Autodesk Fusion 360 part; units mm, degrees
sketch "Sketch1" plane through (0, 0, 0) normal (0, 0, 1) x (1, 0, 0)
  line L0 (0, 0) -> (55, 0)
  line L1 (55, 0) -> (55, 55)
  line L2 (55, 55) -> (0, 55)
  line L3 (0, 55) -> (0, 0)
  circle A0 centre (4, 51) radius 4
  circle A1 centre (51, 51) radius 4
  circle A2 centre (4, 4) radius 4
  circle A3 centre (51, 4) radius 4
  circle A4 centre (4, 51) radius 1.55
  circle A5 centre (51, 51) radius 1.55
  circle A6 centre (4, 4) radius 1.55
  circle A7 centre (51, 4) radius 1.55
  dimension "d1" = 55
  dimension "d2" = 55
  dimension "d3" = 8
  dimension "d4" = 8
  dimension "d5" = 8
  dimension "d6" = 8
  dimension "d7" = 4
  dimension "d8" = 4
  dimension "d9" = 4
  dimension "d10" = 4
  dimension "d11" = 4
  dimension "d12" = 4
  dimension "d13" = 4
  dimension "d14" = 4
  dimension "d15" = 3.1
  dimension "d16" = 3.1
  dimension "d17" = 3.1
  dimension "d18" = 3.1
extrude "Extrude1" add sketch "Sketch1" along normal blind 2 contours L0 L1 L2 L3 A0 A1 A2 A3
extrude "Extrude2" add sketch "Sketch1" along normal blind 4 contours A2 | A3 | A0 | A1
chamfer "Chamfer1" distance 1.8 angle 45 4 edges at (2.5549, 4.5605, 0) (49.5549, 4.5605, 0) (49.5549, 51.5605, 0) (2.5549, 51.5605, 0)
Model file for the job. Use its own axes, mm. A direction names the side the tool comes from. Give positions to 0.01 mm unless a question says otherwise; leave off trailing zeros. Loops run counter-clockwise (first coordinate to the right, second up) from the corner with the lowest first, then second, coordinate; pieces in that order, holes last. Notation, with made-up numbers: M -26,55 L -15,55 A29 ccw -15,81 Z; hole C 48,-4.75 d6. An arc over 180 degrees is marked long. Use one line per item in the form item = value.
Item 1: Two-plate mould, pull along X, no slides. Class faces 3 (the flat face through (0, 28, 1)), 4 (the cylindrical face through (52.846, 54.549, 2.861)), 5 (the flat face through (4, 49, 4)): released by +X, released by -X, zero draft, split by the parting line, or undercut.
Filled in:
face_3 = released by -X
face_4 = undercut
face_5 = zero draft
Item 2: Which spindle directions (+Z, -Z, +X, -X, +Y, -Y) get a long thin tool onto all of the face, cutting with end or side? Do faces 1 (the flat face through (51, 2, 4)), 2 (the flat face through (27, 28, 2)). Say none if no direction does.
Filled in:
face_1 = +Z, +X, -X, +Y, -Y
face_2 = +Z
Item 3: Slice it at A-A on x = 14. List the corners of the cut face in (y, z), and give its area (3 significant figures).
Filled in:
outline = M 0,0 L 55,0 L 55,2 L 0,2 Z
area = 110 mm^2
Item 4: Drill centre lines: L1, parallel to Y at x = 4, z = 3; L2, parallel to X at y = 52, z = 1.3; L3, parallel to X at y = 5, z = 1.45. Where is each one in solid material? Low to high.
Filled in:
L1 = 0 to 2.45, 5.55 to 8, 47 to 49.45, 52.55 to 55
L2 = 0.13 to 2.21, 5.79 to 49.21, 52.79 to 54.87
L3 = 0 to 2.38, 5.62 to 49.38, 52.62 to 55
Item 5: Flat gauge pins, fed straight in: pin 1 Ø1.5 at (x, y) = (38, 30.5) entering from +Z; pin 2 Ø2.5 at (x, y) = (51, 51) entering from +Z (1 decimal). Where does each tip first touch, or does it go through?
Filled in:
pin_1 = 2
pin_2 = through
